The model under review builds one solid part; all positions refer to its coordinate system, in mm. Face numbers are marked on the shaded views. A direction names the side the tool comes from. Round coordinates to 2 decimals unless told otherwise and drop trailing zeros. Order: outer loops, then holes, each group sorted by start corner. A loop starts at its lowest first (then second) coordinate and runs counter-clockwise, first axis right, second up. Notation, with made-up numbers: (73.5, 80.25) - (125.5, 80.25) arc R21 cw to (125.5, 87.25) - close; hole circle Ø5 at (19, -33.75). An arc over 180 degrees is marked (long way). One line per question, with ' | ' between items. Start each with the question number.
Item 1: Add section A-A on y = -23. State how many separate pieces and enclosed holes the cut face has, and give its area (4 significant figures).
Item 2: Add section B-B on x = 58.5. State the section outline as (y, z) points.
Item 3: Tool access review of the marked faces 1 and 2: name each direction out of +Z, -Z, +X, -X, +Y, -Y from which nothing blocks a thin tool from reaching the whole face with its end or side.
Item 4: Insertion check: pin 1 Ø1.1 at (y, z) = (-27.5, 4) entering from +X; pin 2 Ø5 at (x, y) = (50.5, -28) entering from +Z. Each pin has a flat end and moves straight along its axis. Give the tip position at first contact, or say it passes through.
Item 5: For L1, parallel to Z at x = 34, y = -32; L2, parallel to Z at x = 37, y = -4.5; L3, parallel to Z at x = 49.5, y = -26, list the stretches that pass through material, from the lowest coordinate up. Write a range as [from, to].
from build123d import *

# Parameters (mm, degrees)
F0_W     = 69
F0_H     = 45
F0_W_2   = 3
F0_H_2   = 35
F1_DEPTH = 1.1
F3_DEPTH = 45
F4_SIZE  = 0.7
F5_R     = 2


with BuildPart() as f1:
    # F0 (on Top) → F1 (new body)
    with BuildSketch(Plane.XY):
        with Locations((34.5, -22.5)):
            Rectangle(F0_W, F0_H)
        with Locations((13.5, -22.5)):
            Rectangle(F0_W_2, F0_H_2, mode=Mode.SUBTRACT)
        with Locations((19.5, -22.5)):
            Rectangle(F0_W_2, F0_H_2, mode=Mode.SUBTRACT)
        with Locations((25.5, -22.5)):
            Rectangle(F0_W_2, F0_H_2, mode=Mode.SUBTRACT)
        with Locations((31.5, -22.5)):
            Rectangle(F0_W_2, F0_H_2, mode=Mode.SUBTRACT)
        with Locations((37.5, -22.5)):
            Rectangle(F0_W_2, F0_H_2, mode=Mode.SUBTRACT)
        with Locations((43.5, -22.5)):
            Rectangle(F0_W_2, F0_H_2, mode=Mode.SUBTRACT)
        with Locations((49.5, -22.5)):
            Rectangle(F0_W_2, F0_H_2, mode=Mode.SUBTRACT)
        with Locations((55.5, -22.5)):
            Rectangle(F0_W_2, F0_H_2, mode=Mode.SUBTRACT)
    extrude(amount=F1_DEPTH)

    # F2 (on face) → F3 (join, through all)
    with BuildSketch(Plane(origin=(0, 0, 0), x_dir=(-1, 0, 0), z_dir=(0, 1, 0))):
        Polygon((-12, 1.1), (-10.5640519817, 1.1), (-14, 5.1948033947), (-14, 3.4835071852), align=None)
        Polygon((-18, 1.1), (-16.5640519817, 1.1), (-20, 5.1948033947), (-20, 3.4835071852), align=None)
        Polygon((-24, 1.1), (-22.5640519817, 1.1), (-26, 5.1948033947), (-26, 3.4835071852), align=None)
        Polygon((-32, 3.4835071852), (-30, 1.1), (-28.5640519817, 1.1), (-32, 5.1948033947), align=None)
        Polygon((-38, 3.4835071852), (-36, 1.1), (-34.5640519817, 1.1), (-38, 5.1948033947), align=None)
        Polygon((-44, 3.4835071852), (-42, 1.1), (-40.5640519817, 1.1), (-44, 5.1948033947), align=None)
        Polygon((-50, 3.4835071852), (-48, 1.1), (-46.5640519817, 1.1), (-50, 5.1948033947), align=None)
        Polygon((-56, 3.4835071852), (-54, 1.1), (-52.5640519817, 1.1), (-56, 5.1948033947), align=None)
    extrude(amount=-F3_DEPTH)

    # F4
    f4_edges = [f1.edges().sort_by_distance(p)[0] for p in [
        (14, -22.5, 5.194803),
        (20, -22.5, 5.194803),
        (26, -22.5, 5.194803),
        (32, -22.5, 5.194803),
        (38, -22.5, 5.194803),
        (44, -22.5, 5.194803),
        (50, -22.5, 5.194803),
        (56, -22.5, 5.194803),
    ]]
    chamfer(f4_edges, length=F4_SIZE)

    # F5
    f5_edges = [f1.edges().sort_by_distance(p)[0] for p in [
        (25.775024, -45, 4.576688),
        (13.775024, -45, 4.576688),
        (19.775024, -45, 4.576688),
        (31.775024, -45, 4.576688),
        (37.775024, -45, 4.576688),
        (43.775024, -45, 4.576688),
        (49.775024, -45, 4.576688),
        (55.775024, -45, 4.576688),
        (13.775024, 0, 4.576688),
        (19.775024, 0, 4.576688),
        (25.775024, 0, 4.576688),
        (31.775024, 0, 4.576688),
        (37.775024, 0, 4.576688),
        (43.775024, 0, 4.576688),
        (49.775024, 0, 4.576688),
        (55.775024, 0, 4.576688),
    ]]
    fillet(f5_edges, radius=F5_R)


solid = f1.part
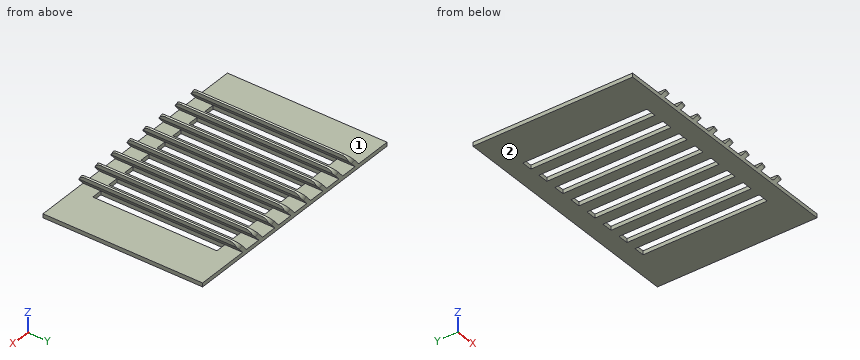
Determined:
1) separate pieces: 9 | enclosed holes: 0 | area: 85.45 mm2
2) outline: (-45, 0) - (0, 0) - (0, 1.1) - (-45, 1.1) - close
3) face 1: +Z, -X, +Y, -Y | face 2: -Z, +X, -X, +Y, -Y
4) pin 1: x = 56 | pin 2: z = 4.66
5) L1: [0, 1.1] | L2: [0, 1.1], [2.29, 4] | L3: [2.89, 4.6]
